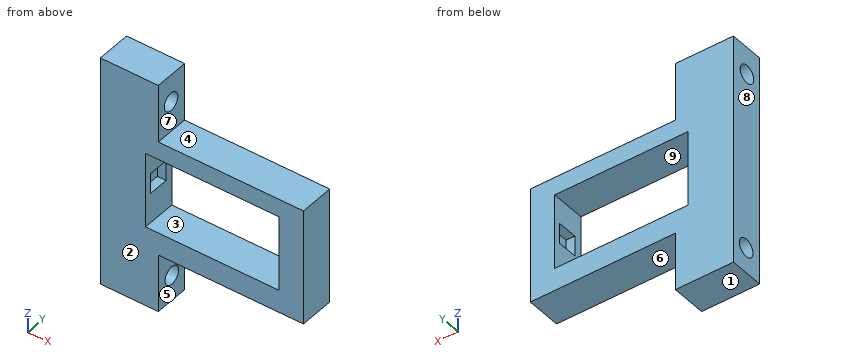
```python
from build123d import *

# Parameters (mm, degrees)
F0_W      = 46
F0_H      = 26
F2_DEPTH  = 12
F4_D      = 6.2
F5_D      = 6.2
F7_W      = 7
F7_H      = 7
F8_DEPTH  = 3
F9_W      = 7
F9_H      = 7
F10_DEPTH = 3


with BuildPart() as f2:
    # F0 (on Front) → F2 (new body)
    with BuildSketch(Plane.XZ):
        Polygon((4.415234, -27.81175), (4.415234, -7.81175), (54.415234, -7.81175), (54.415234, 32.18825), (4.415234, 32.18825), (4.415234, 52.18825), (-15.584766, 52.18825), (-15.584766, -27.81175), align=None)
        with Locations((23, 13)):
            Rectangle(F0_W, F0_H, mode=Mode.SUBTRACT)
    extrude(amount=F2_DEPTH)

    # F4 (through all)
    with Locations(Plane.YZ.offset(25)):
        with Locations((-6.192415, 42.658858)):
            Hole(F4_D / 2)

    # F5 (through all)
    with Locations(Plane.YZ.offset(25)):
        with Locations((-5.817117, -18.983817)):
            Hole(F5_D / 2)

    # F7 (on Right) → F8 (cut)
    with BuildSketch(Plane.YZ):
        with Locations((-6.127085, 13.853554)):
            Rectangle(F7_W, F7_H)
    extrude(amount=-F8_DEPTH, mode=Mode.SUBTRACT)

    # F9 (on offset) → F10 (cut)
    with BuildSketch(Plane.YZ.offset(46)):
        with Locations((-5.657963, 13.853554)):
            Rectangle(F9_W, F9_H)
    extrude(amount=F10_DEPTH, mode=Mode.SUBTRACT)


solid = f2.part
```
Design review of the part built by this model. Coordinates are the model's own, in mm. Face numbers are marked on the shaded views. A direction names the side the tool comes from. Coordinates: 2 decimals unless noted, no trailing zeros. Order: outer loops, then holes, each group sorted by start corner. A loop starts at its lowest first (then second) coordinate and runs counter-clockwise, first axis right, second up. Notation, with made-up numbers: M 49.25,57 L 83.25,57 A27 ccw 83.25,84 Z; hole C -39,61 d8. An arc over 180 degrees is marked long. Answer as a JSON object with one key per item and string values. Group by question number.
1) Tool access review of the marked faces 1, 2, 3, 4 and 5: name each direction out of +Z, -Z, +X, -X, +Y, -Y from which nothing blocks a thin tool from reaching the whole face with its end or side.
2) Add section B-B, the plane z = 15. Write out the cut boundary in (x, y), then the cut area to 3 significant figures.
3) Add section D-D, the plane y = -10.5. Write out the cut boundary in (x, z).
4) Add section A-A, the plane x = 31. Write out the cut boundary in (y, z), then the cut area to 3 significant figures.
5) Wall thickness on L1, parallel to Z at x = 21.5, y = -7; L2, parallel to Z at x = 4, y = -9.5; L3, parallel to X at y = -6, z = 5: over which ranges is each line inside the solid? List them lowest first.
6) Mouldability with a two-part tool opening along X and no side actions: class the marked faces 6, 7, 8 and 9 as pulls with the +X half, pulls with the -X half, needs draft (parallel to the pull), parting line crosses it, or undercut.
7) For pin 1 (1.5 mm diameter, centred on x = -1.5, z = 12.5, fed in from +Y); pin 2 (6 mm diameter, centred on x = 30.5, y = -9, fed in from -Z); pin 3 (3 mm diameter, centred on x = 24, y = -7.5, fed in from +Z), all flat-tipped, find the tip position at first contact; note any pin that passes through.
8) Add section C-C, the plane y = -5.5. Write out the cut boundary in (x, z), then the cut area to 3 significant figures.
Computed values:
{
 "1": {"face 1": "-Z, +X, -X, +Y, -Y", "face 2": "+Z, -Z, +X, -X, -Y", "face 3": "+Y, -Y", "face 4": "+Z, +X, +Y, -Y", "face 5": "-Z, +X, +Y, -Y"},
 "2": {"outline": "M -15.58,-12 L 0,-12 L 0,-9.63 L -3,-9.63 L -3,-2.63 L 0,-2.63 L 0,0 L -15.58,0 Z; M 46,-12 L 54.42,-12 L 54.42,0 L 46,0 L 46,-2.16 L 49,-2.16 L 49,-9.16 L 46,-9.16 Z", "area": "246 mm^2"},
 "3": {"outline": "M -15.58,-27.81 L 4.42,-27.81 L 4.42,-7.81 L 54.42,-7.81 L 54.42,32.19 L 4.42,32.19 L 4.42,52.19 L -15.58,52.19 Z; hole M 0,0 L 46,0 L 46,26 L 0,26 Z"},
 "4": {"outline": "M -12,-7.81 L 0,-7.81 L 0,0 L -12,0 Z; M -12,26 L 0,26 L 0,32.19 L -12,32.19 Z", "area": "168 mm^2"},
 "5": {"L1": "z = -7.81 to 0, 26 to 32.19", "L2": "z = -27.81 to 0, 26 to 52.19", "L3": "x = -15.58 to 0, 46 to 54.42"},
 "6": {"face 6": "needs draft", "face 7": "pulls with the +X half", "face 8": "pulls with the -X half", "face 9": "undercut"},
 "7": {"pin 1": "stops at y = 0", "pin 2": "stops at z = -7.81", "pin 3": "stops at z = 32.19"},
 "8": {"outline": "M -15.58,-27.81 L 4.42,-27.81 L 4.42,-22.07 L -15.58,-22.07 Z; M -15.58,-15.9 L 4.42,-15.9 L 4.42,-7.81 L 54.42,-7.81 L 54.42,32.19 L 4.42,32.19 L 4.42,39.64 L -15.58,39.64 Z; M -15.58,45.68 L 4.42,45.68 L 4.42,52.19 L -15.58,52.19 Z; hole M -3,10.35 L 0,10.35 L 0,0 L 46,0 L 46,10.35 L 49,10.35 L 49,17.35 L 46,17.35 L 46,26 L 0,26 L 0,17.35 L -3,17.35 Z", "area": "2,120 mm^2"}
}
